from build123d import *

# Parameters (mm, degrees)
SKETCH2_W                = 55.53941402
SKETCH2_H                = 35.345852224
BOSS_EXTRUDE1_DEPTH      = 20.066
CONVERT_SOLID10_START    = -25.769706946
CONVERT_SOLID10_DEPTH    = 51.539413892
CONVERT_SOLID10_START_2  = -29
CONVERT_SOLID10_2_DEPTH  = 58
CONVERT_SOLID10_3_DEPTH  = 58
CONVERT_SOLID10_4_DEPTH  = 2.937399826
CONVERT_SOLID10_START_3  = 26.062600174
CONVERT_SOLID10_5_DEPTH  = 2.937399826
CONVERT_SOLID10_START_4  = -26.062600174
CONVERT_SOLID10_6_DEPTH  = 0.292893228
CONVERT_SOLID10_START_5  = 25.769706946
CONVERT_SOLID10_7_DEPTH  = 0.292893228
CONVERT_SOLID10_START_6  = -15.965819276
CONVERT_SOLID10_8_DEPTH  = 31.931638552
CONVERT_SOLID10_9_DEPTH  = 0.292893228
CONVERT_SOLID10_START_7  = 15.672926048
CONVERT_SOLID10_10_DEPTH = 0.292893228


with BuildPart() as part:
    # Sketch2 → Boss-Extrude1 (new body)
    with BuildSketch(Plane(origin=(0, 0, 0), x_dir=(1, 0, 0), z_dir=(0, 1, 0))):
        Rectangle(SKETCH2_W, SKETCH2_H)
    extrude(amount=BOSS_EXTRUDE1_DEPTH)

    # Convert-Solid10: read off the stored shape, not the designer's step
    # Convert-Solid10 outline → Convert-Solid10 (cut)
    with BuildSketch(Plane.YZ.offset(CONVERT_SOLID10_START)):
        with BuildLine():
            Line((0, 16.67292608), (0, -16.67292608))
            Line((0, -16.67292608), (18.065999936, -16.67292608))
            ThreePointArc((18.065999936, -16.67292608), (18.77310674, -16.380032852), (19.065999968, -15.672926048))
            Line((19.065999968, -15.672926048), (19.065999968, 15.672926048))
            ThreePointArc((19.065999968, 15.672926048), (18.77310674, 16.380032852), (18.065999936, 16.67292608))
            Line((18.065999936, 16.67292608), (0, 16.67292608))
        make_face()
    extrude(amount=CONVERT_SOLID10_DEPTH, mode=Mode.SUBTRACT)

    # Convert-Solid10 2 outline → Convert-Solid10 2 (cut)
    with BuildSketch(Plane.YZ.offset(CONVERT_SOLID10_START_2)):
        with BuildLine():
            Line((0, 15.965819276), (17.57580092, 15.965819276))
            Line((17.57580092, 15.965819276), (17.57580092, 15.672926048))
            Line((17.57580092, 15.672926048), (19.065999968, 15.672926048))
            ThreePointArc((19.065999968, 15.672926048), (18.77310674, 16.380032852), (18.065999936, 16.67292608))
            Line((18.065999936, 16.67292608), (0, 16.67292608))
            Line((0, 16.67292608), (0, 15.965819276))
        make_face()
        with BuildLine():
            Line((17.57580092, -15.965819276), (0, -15.965819276))
            Line((0, -15.965819276), (0, -16.67292608))
            Line((0, -16.67292608), (18.065999936, -16.67292608))
            ThreePointArc((18.065999936, -16.67292608), (18.77310674, -16.380032852), (19.065999968, -15.672926048))
            Line((19.065999968, -15.672926048), (17.57580092, -15.672926048))
            Line((17.57580092, -15.672926048), (17.57580092, -15.965819276))
        make_face()
    extrude(amount=CONVERT_SOLID10_2_DEPTH, mode=Mode.SUBTRACT)

    # Convert-Solid10 3 outline → Convert-Solid10 3 (cut)
    with BuildSketch(Plane.YZ.offset(CONVERT_SOLID10_START_2)):
        with BuildLine():
            Line((20.066, 17.672926112), (18.065999936, 17.672926112))
            ThreePointArc((18.065999936, 17.672926112), (19.480213544, 17.087139656), (20.066, 15.672926048))
            Line((20.066, 15.672926048), (20.066, 17.672926112))
        make_face()
        with BuildLine():
            Line((20.066, -17.672926112), (20.066, -15.672926048))
            ThreePointArc((20.066, -15.672926048), (19.480213544, -17.087139656), (18.065999936, -17.672926112))
            Line((18.065999936, -17.672926112), (20.066, -17.672926112))
        make_face()
    extrude(amount=CONVERT_SOLID10_3_DEPTH, mode=Mode.SUBTRACT)

    # Convert-Solid10 4 outline → Convert-Solid10 4 (cut)
    with BuildSketch(Plane.YZ.offset(CONVERT_SOLID10_START_2)):
        with BuildLine():
            Line((0, 16.67292608), (18.065999936, 16.67292608))
            ThreePointArc((18.065999936, 16.67292608), (18.77310674, 16.380032852), (19.065999968, 15.672926048))
            Line((19.065999968, 15.672926048), (20.066, 15.672926048))
            ThreePointArc((20.066, 15.672926048), (19.480213544, 17.087139656), (18.065999936, 17.672926112))
            Line((18.065999936, 17.672926112), (0, 17.672926112))
            Line((0, 17.672926112), (0, 16.67292608))
        make_face()
        with BuildLine():
            ThreePointArc((18.065999936, -17.672926112), (19.480213544, -17.087139656), (20.066, -15.672926048))
            Line((20.066, -15.672926048), (19.065999968, -15.672926048))
            ThreePointArc((19.065999968, -15.672926048), (18.77310674, -16.380032852), (18.065999936, -16.67292608))
            Line((18.065999936, -16.67292608), (0, -16.67292608))
            Line((0, -16.67292608), (0, -17.672926112))
            Line((0, -17.672926112), (18.065999936, -17.672926112))
        make_face()
    extrude(amount=CONVERT_SOLID10_4_DEPTH, mode=Mode.SUBTRACT)

    # Convert-Solid10 5 outline → Convert-Solid10 5 (cut)
    with BuildSketch(Plane.YZ.offset(CONVERT_SOLID10_START_3)):
        with BuildLine():
            Line((0, 16.67292608), (18.065999936, 16.67292608))
            ThreePointArc((18.065999936, 16.67292608), (18.77310674, 16.380032852), (19.065999968, 15.672926048))
            Line((19.065999968, 15.672926048), (20.066, 15.672926048))
            ThreePointArc((20.066, 15.672926048), (19.480213544, 17.087139656), (18.065999936, 17.672926112))
            Line((18.065999936, 17.672926112), (0, 17.672926112))
            Line((0, 17.672926112), (0, 16.67292608))
        make_face()
        with BuildLine():
            ThreePointArc((18.065999936, -17.672926112), (19.480213544, -17.087139656), (20.066, -15.672926048))
            Line((20.066, -15.672926048), (19.065999968, -15.672926048))
            ThreePointArc((19.065999968, -15.672926048), (18.77310674, -16.380032852), (18.065999936, -16.67292608))
            Line((18.065999936, -16.67292608), (0, -16.67292608))
            Line((0, -16.67292608), (0, -17.672926112))
            Line((0, -17.672926112), (18.065999936, -17.672926112))
        make_face()
    extrude(amount=CONVERT_SOLID10_5_DEPTH, mode=Mode.SUBTRACT)

    # Convert-Solid10 6 outline → Convert-Solid10 6 (cut)
    with BuildSketch(Plane.YZ.offset(CONVERT_SOLID10_START_4)):
        with BuildLine():
            Line((17.57580092, 17.672926112), (17.57580092, 16.67292608))
            Line((17.57580092, 16.67292608), (18.065999936, 16.67292608))
            ThreePointArc((18.065999936, 16.67292608), (18.77310674, 16.380032852), (19.065999968, 15.672926048))
            Line((19.065999968, 15.672926048), (20.066, 15.672926048))
            ThreePointArc((20.066, 15.672926048), (19.480213544, 17.087139656), (18.065999936, 17.672926112))
            Line((18.065999936, 17.672926112), (17.57580092, 17.672926112))
        make_face()
        with BuildLine():
            ThreePointArc((18.065999936, -17.672926112), (19.480213544, -17.087139656), (20.066, -15.672926048))
            Line((20.066, -15.672926048), (19.065999968, -15.672926048))
            ThreePointArc((19.065999968, -15.672926048), (18.77310674, -16.380032852), (18.065999936, -16.67292608))
            Line((18.065999936, -16.67292608), (17.57580092, -16.67292608))
            Line((17.57580092, -16.67292608), (17.57580092, -17.672926112))
            Line((17.57580092, -17.672926112), (18.065999936, -17.672926112))
        make_face()
    extrude(amount=CONVERT_SOLID10_6_DEPTH, mode=Mode.SUBTRACT)

    # Convert-Solid10 7 outline → Convert-Solid10 7 (cut)
    with BuildSketch(Plane.YZ.offset(CONVERT_SOLID10_START_5)):
        with BuildLine():
            Line((17.57580092, 17.672926112), (17.57580092, 16.67292608))
            Line((17.57580092, 16.67292608), (18.065999936, 16.67292608))
            ThreePointArc((18.065999936, 16.67292608), (18.77310674, 16.380032852), (19.065999968, 15.672926048))
            Line((19.065999968, 15.672926048), (20.066, 15.672926048))
            ThreePointArc((20.066, 15.672926048), (19.480213544, 17.087139656), (18.065999936, 17.672926112))
            Line((18.065999936, 17.672926112), (17.57580092, 17.672926112))
        make_face()
        with BuildLine():
            ThreePointArc((18.065999936, -17.672926112), (19.480213544, -17.087139656), (20.066, -15.672926048))
            Line((20.066, -15.672926048), (19.065999968, -15.672926048))
            ThreePointArc((19.065999968, -15.672926048), (18.77310674, -16.380032852), (18.065999936, -16.67292608))
            Line((18.065999936, -16.67292608), (17.57580092, -16.67292608))
            Line((17.57580092, -16.67292608), (17.57580092, -17.672926112))
            Line((17.57580092, -17.672926112), (18.065999936, -17.672926112))
        make_face()
    extrude(amount=CONVERT_SOLID10_7_DEPTH, mode=Mode.SUBTRACT)

    # Convert-Solid10 8 outline → Convert-Solid10 8 (cut)
    with BuildSketch(Plane.XY.offset(CONVERT_SOLID10_START_6)):
        with BuildLine():
            Line((-27.76970701, 20.066), (-27.76970701, 18.065999936))
            ThreePointArc((-27.76970701, 18.065999936), (-27.183920554, 19.480213544), (-25.769706946, 20.066))
            Line((-25.769706946, 20.066), (-27.76970701, 20.066))
        make_face()
        with BuildLine():
            Line((27.76970701, 20.066), (25.769706946, 20.066))
            ThreePointArc((25.769706946, 20.066), (27.183920554, 19.480213544), (27.76970701, 18.065999936))
            Line((27.76970701, 18.065999936), (27.76970701, 20.066))
        make_face()
        with BuildLine():
            ThreePointArc((-25.769706946, 19.065999968), (-26.47681375, 18.77310674), (-26.769706978, 18.065999936))
            Line((-26.769706978, 18.065999936), (-26.769706978, 0))
            Line((-26.769706978, 0), (-25.769706946, 0))
            Line((-25.769706946, 0), (-25.769706946, 19.065999968))
        make_face()
        with BuildLine():
            ThreePointArc((26.769706978, 18.065999936), (26.47681375, 18.77310674), (25.769706946, 19.065999968))
            Line((25.769706946, 19.065999968), (25.769706946, 0))
            Line((25.769706946, 0), (26.769706978, 0))
            Line((26.769706978, 0), (26.769706978, 18.065999936))
        make_face()
    extrude(amount=CONVERT_SOLID10_8_DEPTH, mode=Mode.SUBTRACT)

    # Convert-Solid10 9 outline → Convert-Solid10 9 (cut)
    with BuildSketch(Plane.XY.offset(CONVERT_SOLID10_START_6)):
        with BuildLine():
            ThreePointArc((-25.769706946, 20.066), (-27.183920554, 19.480213544), (-27.76970701, 18.065999936))
            Line((-27.76970701, 18.065999936), (-27.76970701, 17.57580092))
            Line((-27.76970701, 17.57580092), (-26.769706978, 17.57580092))
            Line((-26.769706978, 17.57580092), (-26.769706978, 18.065999936))
            ThreePointArc((-26.769706978, 18.065999936), (-26.47681375, 18.77310674), (-25.769706946, 19.065999968))
            Line((-25.769706946, 19.065999968), (-25.769706946, 20.066))
        make_face()
        with BuildLine():
            ThreePointArc((27.76970701, 18.065999936), (27.183920554, 19.480213544), (25.769706946, 20.066))
            Line((25.769706946, 20.066), (25.769706946, 19.065999968))
            ThreePointArc((25.769706946, 19.065999968), (26.47681375, 18.77310674), (26.769706978, 18.065999936))
            Line((26.769706978, 18.065999936), (26.769706978, 17.57580092))
            Line((26.769706978, 17.57580092), (27.76970701, 17.57580092))
            Line((27.76970701, 17.57580092), (27.76970701, 18.065999936))
        make_face()
    extrude(amount=CONVERT_SOLID10_9_DEPTH, mode=Mode.SUBTRACT)

    # Convert-Solid10 10 outline → Convert-Solid10 10 (cut)
    with BuildSketch(Plane.XY.offset(CONVERT_SOLID10_START_7)):
        with BuildLine():
            ThreePointArc((-25.769706946, 20.066), (-27.183920554, 19.480213544), (-27.76970701, 18.065999936))
            Line((-27.76970701, 18.065999936), (-27.76970701, 17.57580092))
            Line((-27.76970701, 17.57580092), (-26.769706978, 17.57580092))
            Line((-26.769706978, 17.57580092), (-26.769706978, 18.065999936))
            ThreePointArc((-26.769706978, 18.065999936), (-26.47681375, 18.77310674), (-25.769706946, 19.065999968))
            Line((-25.769706946, 19.065999968), (-25.769706946, 20.066))
        make_face()
        with BuildLine():
            ThreePointArc((27.76970701, 18.065999936), (27.183920554, 19.480213544), (25.769706946, 20.066))
            Line((25.769706946, 20.066), (25.769706946, 19.065999968))
            ThreePointArc((25.769706946, 19.065999968), (26.47681375, 18.77310674), (26.769706978, 18.065999936))
            Line((26.769706978, 18.065999936), (26.769706978, 17.57580092))
            Line((26.769706978, 17.57580092), (27.76970701, 17.57580092))
            Line((27.76970701, 17.57580092), (27.76970701, 18.065999936))
        make_face()
    extrude(amount=CONVERT_SOLID10_10_DEPTH, mode=Mode.SUBTRACT)


solid = part.part
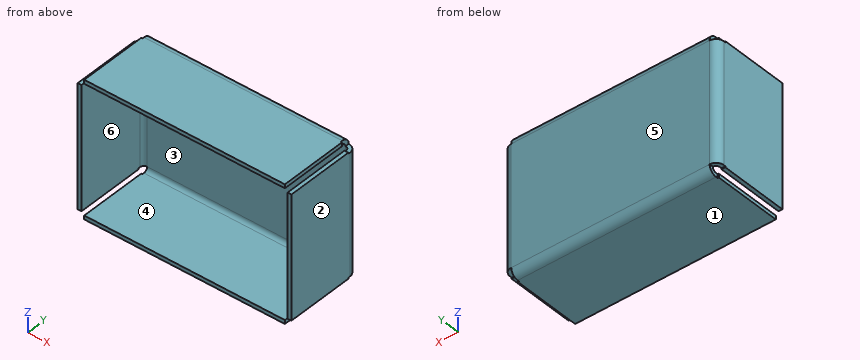
Part model, mm, in its own coordinate system. Face numbers are marked on the shaded views. A direction names the side the tool comes from. Coordinates: 2 decimals unless noted, no trailing zeros. Loops run counter-clockwise (first coordinate to the right, second up) from the corner with the lowest first, then second, coordinate; pieces in that order, holes last. Notation, with made-up numbers: (86, -21) -> (95, -21) arc R15 cw to (95, -8) -> close; hole circle Ø8 at (33.25, -34.5). An arc over 180 degrees is marked (long way). Use a Markdown table: item, result. Add a question column.
Item 1: Which spindle directions (+Z, -Z, +X, -X, +Y, -Y) get a long thin tool onto all of the face, cutting with end or side? Do the marked faces 4, 5 and 6. Say none if no direction does.
Item 2: Probe probe 1 along X at (y, z) = (3.75, -1); probe 2 along Z at (x, y) = (21, 14.25); probe 3 along Y at (x, z) = (0, -6). List the from-to ranges inside material, lowest first.
Item 3: Pull direction X, two halves, no side cores. Call the marked faces 1, 2 and 3: +X half, -X half, draft (parallel to the pull), parting line (faces both ways), or undercut.
Item 4: Band-saw the part on C-C on x = -14.5. Write the cut outline in (y, z).
Item 5: Band-saw the part on B-B on z = 10.5. Write the cut outline in (x, y).
Item 6: Flat gauge pins, fed straight in: P1, Ø0.5, axis at x = -27.5, y = 5.5, coming from the -Z side; P2, Ø5, axis at x = 17, z = 4.5, coming from the -Y side; P3, Ø1, axis at x = -27, y = 19, coming from the +Z side. Where does each tip first touch, or does it go through?
Item 7: Band-saw the part on A-A on y = 2.5. Write the cut outline in (x, z), plus the area to 3 significant figures.
Geometry says:
| question | item | result |
|---|---|---|
| 1 | face 4 | +X, -X, -Y |
| 1 | face 5 | +Z, -Z, +X, -X, +Y |
| 1 | face 6 | +Z, -Z, -Y |
| 2 | probe 1 | -27.77 to -26.77, 26.77 to 27.77 |
| 2 | probe 2 | -17.67 to -16.67, 16.67 to 17.67 |
| 2 | probe 3 | 19.07 to 20.07 |
| 3 | face 1 | draft |
| 3 | face 2 | +X half |
| 3 | face 3 | undercut |
| 4 | outline | (0, -17.67) -> (18.07, -17.67) arc R2 ccw to (20.07, -15.67) -> (20.07, 15.67) arc R2 ccw to (18.07, 17.67) -> (0, 17.67) -> (0, 16.67) -> (18.07, 16.67) arc R1 cw to (19.07, 15.67) -> (19.07, -15.67) arc R1 cw to (18.07, -16.67) -> (0, -16.67) -> close |
| 5 | outline | (-27.77, 0) -> (-26.77, 0) -> (-26.77, 18.07) arc R1 cw to (-25.77, 19.07) -> (25.77, 19.07) arc R1 cw to (26.77, 18.07) -> (26.77, 0) -> (27.77, 0) -> (27.77, 18.07) arc R2 ccw to (25.77, 20.07) -> (-25.77, 20.07) arc R2 ccw to (-27.77, 18.07) -> close |
| 6 | P1 | z = -15.97 |
| 6 | P2 | y = 19.07 |
| 6 | P3 | z = 15.67 |
| 7 | outline | (-27.77, -15.97) -> (-26.77, -15.97) -> (-26.77, 15.97) -> (-27.77, 15.97) -> close; (-26.06, -17.67) -> (26.06, -17.67) -> (26.06, -16.67) -> (-26.06, -16.67) -> close; (-26.06, 16.67) -> (26.06, 16.67) -> (26.06, 17.67) -> (-26.06, 17.67) -> close; (26.77, -15.97) -> (27.77, -15.97) -> (27.77, 15.97) -> (26.77, 15.97) -> close |
| 7 | area | 168 mm² |
